Verification items for this drawing (mm, ordinates from the low corner). Round coordinates to 2 decimals unless told otherwise and drop trailing zeros. Loops run counter-clockwise (first coordinate to the right, second up) from the corner with the lowest first, then second, coordinate; pieces in that order, holes last. Notation, with made-up numbers: (57.5, 13.25) -> (115.5, 13.25) arc R11 ccw to (115.5, 29.25) -> close; hole circle Ø11 at (38, 84). An arc over 180 degrees is marked (long way). One line per question, with ' | ' between items.
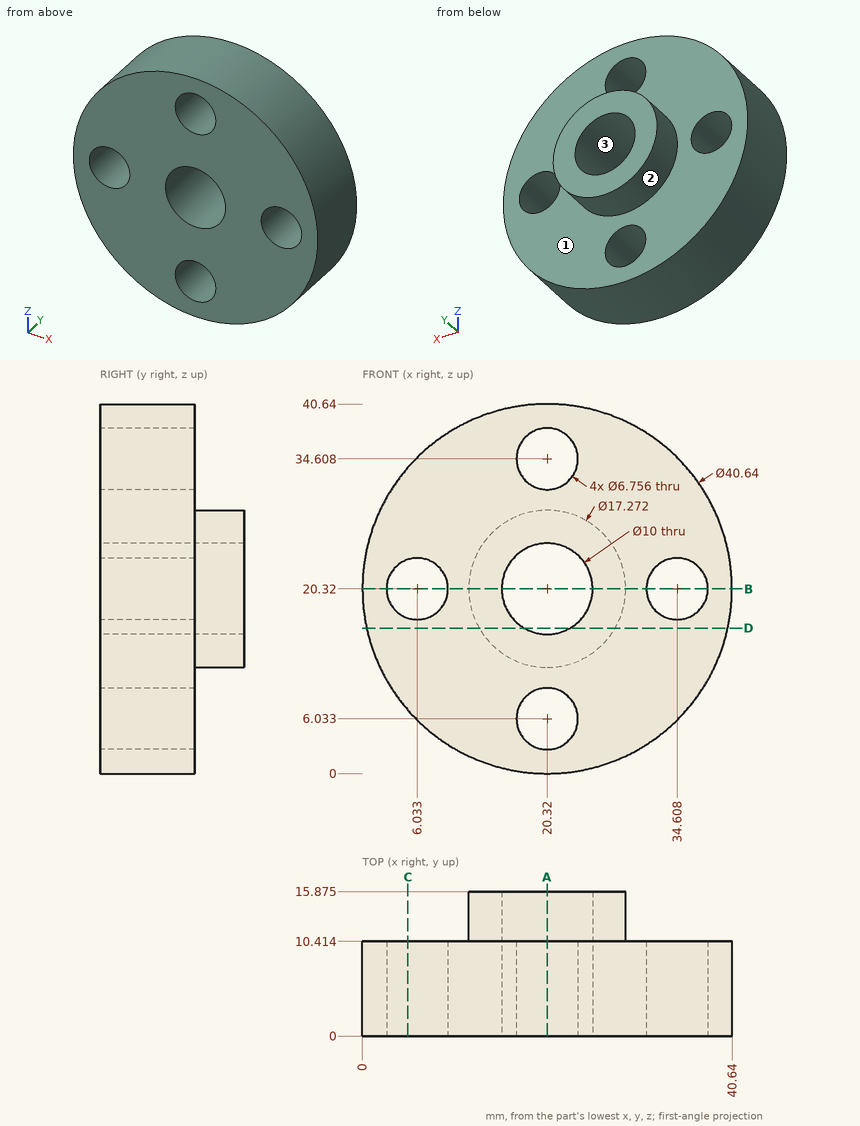
(1) Mould release check, pull along Z, two halves, no side actions. Record for the marked faces 1, 2 and 3: +Z half, -Z half, draft (parallel to the pull), parting line (faces both ways), or undercut.
Answer:
face 1: draft | face 2: parting line | face 3: undercut
(2) Sectioned sample at B-B, the plane z = 20.32. Record the cut outline in (x, y) (1 decimal), and give its area (3 significant figures).
Answer:
outline: (0, 0) -> (2.7, 0) -> (2.7, 10.4) -> (0, 10.4) -> close; (9.4, 0) -> (15.3, 0) -> (15.3, 15.9) -> (11.7, 15.9) -> (11.7, 10.4) -> (9.4, 10.4) -> close; (25.3, 0) -> (31.2, 0) -> (31.2, 10.4) -> (29, 10.4) -> (29, 15.9) -> (25.3, 15.9) -> close; (38, 0) -> (40.6, 0) -> (40.6, 10.4) -> (38, 10.4) -> close | area: 218 mm2
(3) Sectioned sample at D-D, the plane z = 16. Record the cut outline in (x, y) (1 decimal).
Answer:
outline: (0.5, 0) -> (17.8, 0) -> (17.8, 15.9) -> (12.8, 15.9) -> (12.8, 10.4) -> (0.5, 10.4) -> close; (22.8, 0) -> (40.2, 0) -> (40.2, 10.4) -> (27.8, 10.4) -> (27.8, 15.9) -> (22.8, 15.9) -> close
(4) Sectioned sample at C-C, the plane x = 5. Record the cut outline in (y, z) (1 decimal), and give its area (3 significant figures).
Answer:
outline: (0, 7) -> (10.4, 7) -> (10.4, 17.1) -> (0, 17.1) -> close; (0, 23.5) -> (10.4, 23.5) -> (10.4, 33.7) -> (0, 33.7) -> close | area: 211 mm2
(5) Go/stop test with flat-tipped pins: pin 1 (3 mm diameter, centred on x = 33, y = 8.5, fed in from -Z); pin 2 (11 mm diameter, centred on x = 20.32, z = 34.61, fed in from -Y); pin 3 (1.5 mm diameter, centred on y = 7, z = 21.5, fed in from -X) (1 decimal); pin 4 (1.5 mm diameter, centred on y = 13.5, z = 13, fed in from +X) (1 decimal). Record where each tip stops, or that it passes through.
Answer:
pin 1: stops at z = 3.35 | pin 2: stops at y = 0 | pin 3: stops at x = 0 | pin 4: stops at x = 25.9
(6) Sectioned sample at A-A, the plane x = 20.32. Record the cut outline in (y, z) (1 decimal), and give its area (3 significant figures).
Answer:
outline: (0, 0) -> (10.4, 0) -> (10.4, 2.7) -> (0, 2.7) -> close; (0, 9.4) -> (10.4, 9.4) -> (10.4, 11.7) -> (15.9, 11.7) -> (15.9, 15.3) -> (0, 15.3) -> close; (0, 25.3) -> (15.9, 25.3) -> (15.9, 29) -> (10.4, 29) -> (10.4, 31.2) -> (0, 31.2) -> close; (0, 38) -> (10.4, 38) -> (10.4, 40.6) -> (0, 40.6) -> close | area: 218 mm2
(7) Scan lines: probe 1 along X at (y, z) = (4, 20.32) (1 decimal); probe 2 along X at (y, z) = (11.5, 20); probe 3 along Y at (x, z) = (27.5, 5.5) (1 decimal). Record each from-to range of solid material in increasing order.
Answer:
probe 1: x = 0 to 2.7, 9.4 to 15.3, 25.3 to 31.2, 38 to 40.6 | probe 2: x = 11.69 to 15.33, 25.31 to 28.95 | probe 3: y = 0 to 10.4
